The listing builds one solid part. Answer for the finished solid, in the listing's coordinates (mm). Face numbers are marked on the shaded views. Coordinates: 2 decimals unless noted, no trailing zeros. Write each loop counter-clockwise with the first axis right and the second up, starting at its lowest first coordinate (ties: lowest second). Pieces come first, ordered by that corner, then holes.
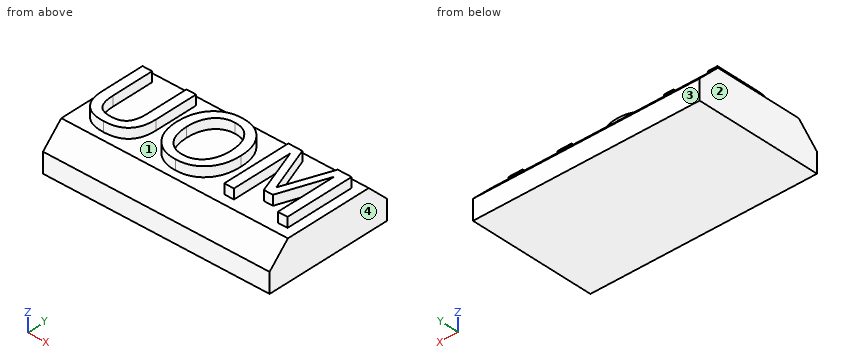
from build123d import *

# Parameters (mm, degrees)
BOSS_EXTRUDE5_DEPTH = 11.427281
BOSS_EXTRUDE6_DEPTH = 0.5


with BuildPart() as part:
    # Sketch6 → Boss-Extrude5 (new body)
    with BuildSketch(Plane(origin=(0, 0, 0), x_dir=(0, 0, -1), z_dir=(1, 0, 0))):
        Polygon((1, 4.929146991), (2, 4.929146991), (2, -1.486632629), (1, -1.486632629), (0, -0.486632629), (0, 3.929146991), align=None)
    extrude(amount=BOSS_EXTRUDE5_DEPTH)

    # Sketch3 → Boss-Extrude6 (add)
    # profile 1 of 3: a face of its own
    with BuildSketch(Plane.XY):
        with BuildLine():
            Line((0.416143204, 3.499962788), (0.903484976, 3.499962788))
            Line((0.903484976, 3.499962788), (0.903484976, 1.371996016))
            add(Edge.make_bspline(
                [(0.903484976, 1.371996016), (0.904227086, 1.326524703), (0.905656325, 1.238950888), (0.914351034, 1.112472094), (0.929908885, 0.995823754), (0.952901435, 0.88903938), (0.980924682, 0.791621238), (1.015086709, 0.703774074), (1.056939832, 0.626271366), (1.104984797, 0.558086727), (1.160610571, 0.498806201), (1.224233651, 0.448193549), (1.295415202, 0.404639357), (1.375404867, 0.37044697), (1.462695851, 0.342558961), (1.558111742, 0.323476327), (1.661242149, 0.312624163), (1.732539226, 0.310954566), (1.769485767, 0.310089371)],
                knots=[0, 0, 0, 0, 1.376819889, 2.651635969, 3.836347594, 4.936722514, 5.955940511, 6.903042086, 7.784610942, 8.616290434, 9.4219432, 10.237023, 11.070988377, 11.94071121, 12.864328567, 13.841290783, 14.88134492, 16, 16, 16, 16], degree=3))
            add(Edge.make_bspline(
                [(1.769485767, 0.310089371), (1.806202381, 0.310952028), (1.877040741, 0.312616375), (1.979473884, 0.323496618), (2.074016457, 0.342434724), (2.160317672, 0.37056602), (2.239557597, 0.404801908), (2.310591352, 0.448180089), (2.374204682, 0.498809996), (2.42983769, 0.558084657), (2.477862395, 0.62627603), (2.519795758, 0.703755997), (2.553648868, 0.791757514), (2.583057817, 0.888807287), (2.604576184, 0.995949131), (2.620568037, 1.112448839), (2.62913327, 1.238957439), (2.630581241, 1.326526942), (2.631333077, 1.371996016)],
                knots=[0, 0, 0, 0, 1.114454679, 2.150147657, 3.122692882, 4.035279244, 4.900768316, 5.736820227, 6.553939311, 7.361607774, 8.195368082, 9.079142573, 10.028613743, 11.052372373, 12.154054081, 13.341729787, 14.619735386, 16, 16, 16, 16], degree=3))
            Line((2.631333077, 1.371996016), (2.631333077, 3.499962788))
            Line((2.631333077, 3.499962788), (3.118674849, 3.499962788))
            Line((3.118674849, 3.499962788), (3.118674849, 1.302771333))
            add(Edge.make_bspline(
                [(3.118674849, 1.302771333), (3.117632966, 1.247119199), (3.115609542, 1.139038072), (3.099395772, 0.982162679), (3.073760625, 0.835658607), (3.03631439, 0.699523534), (2.987830531, 0.574188519), (2.929913308, 0.458712614), (2.859816087, 0.354574755), (2.77943465, 0.260926992), (2.688738665, 0.177698385), (2.587499929, 0.10602186), (2.475912337, 0.045485903), (2.353984334, -0.003248427), (2.222507035, -0.042549241), (2.080438371, -0.068601387), (1.92843276, -0.085798259), (1.82353189, -0.087676906), (1.769485767, -0.088644806)],
                knots=[0, 0, 0, 0, 1.203396059, 2.33709643, 3.407052704, 4.416843994, 5.385341086, 6.309356336, 7.204900642, 8.093184639, 8.972733791, 9.860358641, 10.769263838, 11.711760021, 12.695515199, 13.732034436, 14.831518306, 16, 16, 16, 16], degree=3))
            add(Edge.make_bspline(
                [(1.769485767, -0.088644806), (1.71521014, -0.087673568), (1.609851426, -0.085788222), (1.457142055, -0.068631325), (1.314216014, -0.042395163), (1.181883322, -0.003559879), (1.059492843, 0.045718996), (0.947387007, 0.105755521), (0.846109761, 0.177988639), (0.75466648, 0.26044674), (0.675027309, 0.354825839), (0.605047005, 0.458877246), (0.545964542, 0.573840725), (0.498766704, 0.699718527), (0.460974682, 0.835625191), (0.435446342, 0.982172396), (0.419201909, 1.139035406), (0.417182842, 1.247118293), (0.416143204, 1.302771333)],
                knots=[0, 0, 0, 0, 1.171292133, 2.273687844, 3.313177071, 4.30466322, 5.245410695, 6.15700884, 7.042986791, 7.924584801, 8.807982338, 9.70186505, 10.626436486, 11.59135102, 12.599268744, 13.66723982, 14.798836723, 16, 16, 16, 16], degree=3))
            Line((0.416143204, 1.302771333), (0.416143204, 3.499962788))
        make_face()
    # profile 2 of 3: a face of its own
    with BuildSketch(Plane.XY):
        with BuildLine():
            add(Edge.make_bspline(
                [(5.402397159, 3.544266586), (5.462246122, 3.542948612), (5.579200043, 3.540373092), (5.749821524, 3.516018599), (5.911346929, 3.477588836), (6.063839721, 3.423299268), (6.207501548, 3.35408974), (6.341090707, 3.26794254), (6.465977946, 3.167203043), (6.57950417, 3.050514604), (6.682793918, 2.922216447), (6.772480012, 2.781879471), (6.848877785, 2.63150278), (6.910413596, 2.47007031), (6.959107704, 2.298965057), (6.992313654, 2.116961877), (7.013739577, 1.924922192), (7.016166669, 1.793172801), (7.017409026, 1.725734149)],
                knots=[0, 0, 0, 0, 1.046974495, 2.045946433, 3.009842023, 3.948749427, 4.873574893, 5.794485429, 6.724850033, 7.675874877, 8.638390309, 9.602979465, 10.585554, 11.585350169, 12.622203588, 13.694728314, 14.819998983, 16, 16, 16, 16], degree=3))
            add(Edge.make_bspline(
                [(7.017409026, 1.725734149), (7.016183724, 1.658523681), (7.013794306, 1.527459035), (6.992167411, 1.336142779), (6.959242213, 1.154771949), (6.910243582, 0.9839908), (6.849074922, 0.822869328), (6.772280141, 0.672915871), (6.682784418, 0.532734916), (6.579732711, 0.404417634), (6.465733721, 0.288426434), (6.34111492, 0.187668849), (6.20751823, 0.101465273), (6.063677323, 0.032569648), (5.911610665, -0.023084389), (5.749686437, -0.060093933), (5.579221976, -0.084834545), (5.462253547, -0.087355008), (5.402397159, -0.088644806)],
                knots=[0, 0, 0, 0, 1.177584306, 2.296363576, 3.370365481, 4.404756482, 5.405929662, 6.386251896, 7.352169572, 8.316010668, 9.265464185, 10.197110173, 11.11928907, 12.045388291, 12.986953489, 13.951235703, 14.951583516, 16, 16, 16, 16], degree=3))
            add(Edge.make_bspline(
                [(5.402397159, -0.088644806), (5.342559768, -0.087243888), (5.22565973, -0.084507014), (5.054907212, -0.06132131), (4.893466487, -0.022581169), (4.740913242, 0.031549646), (4.597373281, 0.101113043), (4.463019213, 0.186195092), (4.337474868, 0.286312005), (4.223239698, 0.402297965), (4.119135691, 0.530036826), (4.028797089, 0.669763824), (3.953338421, 0.820478357), (3.890768592, 0.981010653), (3.842305583, 1.152335357), (3.808156093, 1.334197343), (3.786955336, 1.526557072), (3.784492477, 1.65829921), (3.783231811, 1.725734149)],
                knots=[0, 0, 0, 0, 1.046993163, 2.04543576, 3.009348536, 3.94827268, 4.873114636, 5.795280634, 6.726275263, 7.67728276, 8.639205072, 9.605998851, 10.583164017, 11.584437137, 12.617423858, 13.694687211, 14.819977944, 16, 16, 16, 16], degree=3))
            add(Edge.make_bspline(
                [(3.783231811, 1.725734149), (3.784499678, 1.793167465), (3.786976606, 1.924906431), (3.808052274, 2.117063164), (3.842532146, 2.298844092), (3.890587304, 2.4702857), (3.953548456, 2.63111657), (4.028558923, 2.782292585), (4.119360297, 2.922184769), (4.223197774, 3.050551981), (4.337458654, 3.167215801), (4.463016032, 3.267978548), (4.597174521, 3.353910321), (4.740938987, 3.42332509), (4.893451716, 3.477581678), (5.054971582, 3.516020604), (5.2255946, 3.540372555), (5.342548306, 3.54294843), (5.402397159, 3.544266586)],
                knots=[0, 0, 0, 0, 1.178933409, 2.303185988, 3.375492215, 4.41140754, 5.41175692, 6.391624662, 7.35752651, 8.321699006, 9.274695168, 10.207356909, 11.130834481, 12.05482321, 12.992881136, 13.95590464, 14.953972757, 16, 16, 16, 16], degree=3))
        make_face()
        with BuildLine():
            add(Edge.make_bspline(
                [(5.400320419, 3.145532409), (5.35803641, 3.14427069), (5.27541253, 3.141805264), (5.154622477, 3.124415503), (5.040796804, 3.094770228), (4.933403863, 3.052757792), (4.833088358, 2.998703881), (4.739097158, 2.932857447), (4.652403926, 2.854815258), (4.572869424, 2.765379259), (4.501719741, 2.665767382), (4.440079646, 2.55698884), (4.386908752, 2.439945508), (4.344436085, 2.313670722), (4.311169081, 2.178899707), (4.288130717, 2.035568821), (4.273106925, 1.883655163), (4.271432966, 1.779305484), (4.270573583, 1.725734149)],
                knots=[0, 0, 0, 0, 0.992078402, 1.938542973, 2.856561574, 3.746427499, 4.637939252, 5.524223217, 6.432997522, 7.368745408, 8.327383014, 9.299866671, 10.29827865, 11.339356729, 12.421474065, 13.551982278, 14.743229712, 16, 16, 16, 16], degree=3))
            add(Edge.make_bspline(
                [(4.270573583, 1.725734149), (4.271435175, 1.672623784), (4.273116806, 1.568964413), (4.288197128, 1.417753347), (4.311085619, 1.274857783), (4.344420664, 1.140549714), (4.387052766, 1.014803381), (4.440069416, 0.897940197), (4.501709798, 0.789146996), (4.57291796, 0.689609896), (4.652124511, 0.600014393), (4.739595317, 0.522951233), (4.832626534, 0.455951117), (4.933648368, 0.403070886), (5.040757185, 0.360783207), (5.154633534, 0.33122535), (5.275409573, 0.313811414), (5.358035409, 0.311349362), (5.400320419, 0.310089371)],
                knots=[0, 0, 0, 0, 1.248257537, 2.436315255, 3.568920878, 4.647780726, 5.68565685, 6.685921162, 7.660209049, 8.620625195, 9.558109156, 10.4649585, 11.356013141, 12.24662183, 13.138138705, 14.057860487, 15.006081015, 16, 16, 16, 16], degree=3))
            add(Edge.make_bspline(
                [(5.400320419, 0.310089371), (5.442604788, 0.311350447), (5.525229374, 0.313814618), (5.646014372, 0.331213368), (5.759858322, 0.36082614), (5.866893881, 0.402841381), (5.967484462, 0.456415555), (6.060976588, 0.522453192), (6.147787085, 0.600316817), (6.227118702, 0.689535237), (6.298104952, 0.789362494), (6.360719863, 0.897721104), (6.413532899, 1.014835582), (6.45623582, 1.140540581), (6.48955073, 1.274860403), (6.512444996, 1.417752597), (6.527523684, 1.568964615), (6.529205545, 1.672623853), (6.530067254, 1.725734149)],
                knots=[0, 0, 0, 0, 0.994024979, 1.942346626, 2.862166489, 3.753778437, 4.639694184, 5.535275203, 6.438171751, 7.375755687, 8.336274254, 9.313365839, 10.313736821, 11.351723626, 12.430698526, 13.563424932, 14.751609347, 16, 16, 16, 16], degree=3))
            add(Edge.make_bspline(
                [(6.530067254, 1.725734149), (6.529207753, 1.779305414), (6.527533561, 1.883654958), (6.512511413, 2.035569575), (6.489467259, 2.178897083), (6.456220518, 2.313679923), (6.41367661, 2.439913134), (6.360709572, 2.557207896), (6.298094939, 2.665551865), (6.22716738, 2.76545382), (6.147506692, 2.854513751), (6.061474862, 2.933355261), (5.967022545, 2.998239032), (5.867139571, 3.052987268), (5.759818468, 3.094727141), (5.646025495, 3.124427529), (5.525226399, 3.141802048), (5.442603781, 3.144269602), (5.400320419, 3.145532409)],
                knots=[0, 0, 0, 0, 1.256900501, 2.448271359, 3.578896704, 4.661126157, 5.702312102, 6.700827525, 7.676106732, 8.634843661, 9.5706885, 10.475531073, 11.366345495, 12.253184336, 13.14314246, 14.061256176, 15.007818809, 16, 16, 16, 16], degree=3))
        make_face(mode=Mode.SUBTRACT)
    # profile 3 of 3: a face of its own
    with BuildSketch(Plane.XY):
        Polygon((7.770573583, 3.499962788), (8.475973109, 3.499962788), (9.363433552, 1.116556934), (10.259893204, 3.499962788), (10.960447001, 3.499962788), (10.960447001, -3.7212e-05), (10.473105229, -3.7212e-05), (10.473105229, 3.072846491), (9.595336242, 0.680441428), (9.135684343, 0.680441428), (8.257915355, 3.072846491), (8.257915355, -3.7212e-05), (7.770573583, -3.7212e-05), align=None)
    extrude(amount=BOSS_EXTRUDE6_DEPTH)


solid = part.part
1. Find the intervals of material crossed by L1, parallel to X at y = 0.25, z = 0.1; L2, parallel to Z at x = 7.75, y = -0.25; L3, parallel to X at y = 0.5, z = 0.05, in increasing order.
Results found:
L1: x = 0.77 to 2.77, 4.38 to 6.42, 7.77 to 8.26, 10.47 to 10.96
L2: z = -2 to 0
L3: x = 0.58 to 1.16, 2.37 to 2.95, 4.15 to 4.77, 6.03 to 6.65, 7.77 to 8.26, 10.47 to 10.96
2. For a pull along X with two mould halves and no side action, classify the marked faces 1, 2, 3 and 4 as pulls with the +X half, pulls with the -X half, needs draft (parallel to the pull), parting line crosses it, or undercut.
Results found:
face 1: undercut
face 2: pulls with the -X half
face 3: needs draft
face 4: pulls with the +X half
3. Section B-B on x = 10.75 is taken. Give the vertices of the cut face in (y, z), then the cut area to 3 significant figures.
Results found:
outline: (-1.49, -2) - (4.93, -2) - (4.93, -1) - (3.93, 0) - (3.5, 0) - (3.5, 0.5) - (0, 0.5) - (0, 0) - (-0.49, 0) - (-1.49, -1) - close
area: 13.6 mm2
4. Section D-D on z = -0.7 is taken. Give the vertices of the cut face in (x, y), then the cut area to 3 significant figures.
Results found:
outline: (0, -1.19) - (11.43, -1.19) - (11.43, 4.63) - (0, 4.63) - close
area: 66.5 mm2
5. Section A-A on z = 0.2 is taken. State how many separate pieces and enclosed holes the cut face has, then the cut area to 3 significant figures.
Results found:
separate pieces: 3
enclosed holes: 1
area: 13.6 mm2
6. Flat-ended cylindrical pins translate along their axes: P1, Ø0.5, axis at x = 0.5, z = 0.5, coming from the +Y side; P2, Ø0.6, axis at y = 2.5, z = 0.5, coming from the +X side; P3, Ø0.6, axis at x = 8, z = 0, coming from the +Y side. Find the tip coordinate at first contact, or state that the pin passes through.
Results found:
P1: stops at y = 3.5
P2: stops at x = 10.96
P3: stops at y = 4.23
7. Section C-C on x = 3.25 is taken. Give the vertices of the cut face in (y, z), then the cut area to 3 significant figures.
Results found:
outline: (-1.49, -2) - (4.93, -2) - (4.93, -1) - (3.93, 0) - (-0.49, 0) - (-1.49, -1) - close
area: 11.8 mm2
